```python
from build123d import *

# Parameters (mm, degrees)
SKETCH_1_R          = 1.5
EXTRUDE_1_DEPTH     = 10
CUT_EXTRUDE_2_DEPTH = 10


with BuildPart() as part:
    # 草图1 → 凸台-拉伸1 (new body)
    with BuildSketch(Plane.XY):
        with BuildLine():
            Line((1.5, 19.943670675), (1.5, 25))
            Line((1.5, 25), (-1.5, 25))
            Line((-1.5, 25), (-1.5, 19.943670675))
            ThreePointArc((-1.5, 19.943670675), (-6.180339888, 19.021130326), (-10.509070008, 17.016446385))
            Line((-10.509070008, 17.016446385), (-13.481105816, 21.107102738))
            Line((-13.481105816, 21.107102738), (-15.908156799, 19.343746981))
            Line((-15.908156799, 19.343746981), (-12.936120991, 15.253090628))
            ThreePointArc((-12.936120991, 15.253090628), (-16.180339887, 11.755705046), (-18.504032463, 7.589517943))
            Line((-18.504032463, 7.589517943), (-23.312887416, 9.152009634))
            Line((-23.312887416, 9.152009634), (-24.239938399, 6.298840085))
            Line((-24.239938399, 6.298840085), (-19.431083446, 4.736348394))
            ThreePointArc((-19.431083446, 4.736348394), (-20, 0), (-19.431083446, -4.736348394))
            Line((-19.431083446, -4.736348394), (-24.239938399, -6.298840085))
            Line((-24.239938399, -6.298840085), (-23.312887416, -9.152009634))
            Line((-23.312887416, -9.152009634), (-18.504032463, -7.589517943))
            ThreePointArc((-18.504032463, -7.589517943), (-16.180339887, -11.755705046), (-12.936120991, -15.253090628))
            Line((-12.936120991, -15.253090628), (-15.908156799, -19.343746981))
            Line((-15.908156799, -19.343746981), (-13.481105816, -21.107102738))
            Line((-13.481105816, -21.107102738), (-10.509070008, -17.016446385))
            ThreePointArc((-10.509070008, -17.016446385), (-6.180339887, -19.021130326), (-1.5, -19.943670675))
            Line((-1.5, -19.943670675), (-1.5, -25))
            Line((-1.5, -25), (1.5, -25))
            Line((1.5, -25), (1.5, -19.943670675))
            ThreePointArc((1.5, -19.943670675), (6.180339888, -19.021130326), (10.509070008, -17.016446385))
            Line((10.509070008, -17.016446385), (13.481105816, -21.107102738))
            Line((13.481105816, -21.107102738), (15.908156799, -19.343746981))
            Line((15.908156799, -19.343746981), (12.936120991, -15.253090628))
            ThreePointArc((12.936120991, -15.253090628), (16.180339887, -11.755705046), (18.504032463, -7.589517943))
            Line((18.504032463, -7.589517943), (23.312887416, -9.152009634))
            Line((23.312887416, -9.152009634), (24.239938399, -6.298840085))
            Line((24.239938399, -6.298840085), (19.431083446, -4.736348394))
            ThreePointArc((19.431083446, -4.736348394), (20, 0), (19.431083446, 4.736348394))
            Line((19.431083446, 4.736348394), (24.239938399, 6.298840085))
            Line((24.239938399, 6.298840085), (23.312887416, 9.152009634))
            Line((23.312887416, 9.152009634), (18.504032463, 7.589517943))
            ThreePointArc((18.504032463, 7.589517943), (16.180339887, 11.755705046), (12.936120991, 15.253090628))
            Line((12.936120991, 15.253090628), (15.908156799, 19.343746981))
            Line((15.908156799, 19.343746981), (13.481105816, 21.107102738))
            Line((13.481105816, 21.107102738), (10.509070008, 17.016446385))
            ThreePointArc((10.509070008, 17.016446385), (6.180339887, 19.021130326), (1.5, 19.943670675))
        make_face()
        with Locations((0, 12.5)):
            Circle(SKETCH_1_R, mode=Mode.SUBTRACT)
        with Locations((10.825317547, -6.25)):
            Circle(SKETCH_1_R, mode=Mode.SUBTRACT)
        with Locations((-10.825317547, -6.25)):
            Circle(SKETCH_1_R, mode=Mode.SUBTRACT)
    extrude(amount=EXTRUDE_1_DEPTH)

    # 草图2 → 切除-拉伸2 (cut)
    with BuildSketch(Plane.XY):
        with BuildLine():
            Line((-9.312271895, 3.644391878), (-13.675265955, 6.163367673))
            ThreePointArc((-13.675265955, 6.163367673), (-14.883992786, 1.861923398), (-14.772116295, -2.604722665))
            Line((-14.772116295, -2.604722665), (-17.726539554, -3.125667198))
            ThreePointArc((-17.726539554, -3.125667198), (-15.588457268, 9), (-6.15636258, 16.914467174))
            Line((-6.15636258, 16.914467174), (-5.13030215, 14.095389312))
            ThreePointArc((-5.13030215, 14.095389312), (-9.054469356, 11.958954164), (-12.175265955, 8.761443884))
            Line((-12.175265955, 8.761443884), (-7.812271895, 6.242468089))
            ThreePointArc((-7.812271895, 6.242468089), (0, 10), (7.812271895, 6.242468089))
            Line((7.812271895, 6.242468089), (12.175265955, 8.761443884))
            ThreePointArc((12.175265955, 8.761443884), (9.054469356, 11.958954164), (5.13030215, 14.095389312))
            Line((5.13030215, 14.095389312), (6.15636258, 16.914467174))
            ThreePointArc((6.15636258, 16.914467174), (15.588457268, 9), (17.726539554, -3.125667198))
            Line((17.726539554, -3.125667198), (14.772116295, -2.604722665))
            ThreePointArc((14.772116295, -2.604722665), (14.883992786, 1.861923398), (13.675265955, 6.163367673))
            Line((13.675265955, 6.163367673), (9.312271895, 3.644391878))
            ThreePointArc((9.312271895, 3.644391878), (8.660254038, -5), (1.5, -9.886859967))
            Line((1.5, -9.886859967), (1.5, -14.924811557))
            ThreePointArc((1.5, -14.924811557), (5.829523431, -13.820877562), (9.641814145, -11.490666647))
            Line((9.641814145, -11.490666647), (11.570176974, -13.788799976))
            ThreePointArc((11.570176974, -13.788799976), (0, -18), (-11.570176974, -13.788799976))
            Line((-11.570176974, -13.788799976), (-9.641814145, -11.490666647))
            ThreePointArc((-9.641814145, -11.490666647), (-5.829523431, -13.820877562), (-1.5, -14.924811557))
            Line((-1.5, -14.924811557), (-1.5, -9.886859967))
            ThreePointArc((-1.5, -9.886859967), (-8.660254038, -5), (-9.312271895, 3.644391878))
        make_face()
    extrude(amount=CUT_EXTRUDE_2_DEPTH, mode=Mode.SUBTRACT)


solid = part.part
```
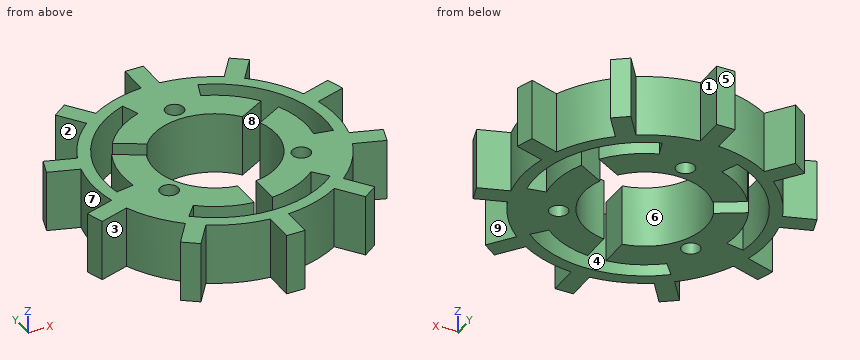
Verification items for the finished model (mm, model axes). Face numbers are marked on the shaded views. A direction names the side the tool comes from. Round coordinates to 2 decimals unless told otherwise and drop trailing zeros. Write each loop counter-clockwise with the first axis right and the second up, starting at its lowest first coordinate (ties: lowest second). Pieces come first, ordered by that corner, then holes. Notation, with made-up numbers: (-28.5, 89) -> (24.5, 89) arc R8 ccw to (24.5, 97) -> close; hole circle Ø10 at (35.5, 48.5). An arc over 180 degrees is marked (long way). Write each question's results on one line, items separated by ' | '. Start each with the question number.
1. Cross-section at C-C (x = 0). Enter the section's corners in (y, z), then the cut area to 3 significant figures.
2. Depth check by flat-ended pin: P1, Ø6, axis at x = -19, z = 6, coming from the -Y side; P2, Ø4, axis at y = 21.5, z = 5.5, coming from the -X side; P3, Ø5.5, axis at y = -12.5, z = 7.5, coming from the +X side; P4, Ø6, axis at x = -4, z = 3, coming from the -Y side. Enter the tip coordinate at first touch or a pass-through.
3. Cross-section at D-D (z = 3.75). Count the separate pieces of the cut face and the enclosed holes in it, then the cut area to 3 significant figures.
4. Set-up check for the marked faces 1, 2, 3, 4 and 5: record each of +Z, -Z, +X, -X, +Y, -Y from which the full face is reachable in a straight line by a thin tool's end or side.
5. Material ranges on probe 1 along X at (y, z) = (-21, 4.5); probe 2 along Y at (x, z) = (12, 4.25); probe 3 along Y at (x, z) = (-2, 3), recorded low to high. Write a range as from..to.
6. Cross-section at A-A (x = -8.5). Enter the section's corners in (y, z).
7. Draft check along X on the marked faces 6, 7, 8 and 9. Enter one of: +X half, -X half, draft (parallel to the pull), parting line (faces both ways), or undercut.
8. Cross-section at B-B (y = -7). Enter the section's corners in (x, z), then the cut area to 3 significant figures.
Solutions:
1) outline: (-25, 0) -> (-18, 0) -> (-18, 10) -> (-25, 10) -> close; (10, 0) -> (11, 0) -> (11, 10) -> (10, 10) -> close; (14, 0) -> (25, 0) -> (25, 10) -> (14, 10) -> close | area: 190 mm2
2) P1: stops at y = -12 | P2: stops at x = -15.69 | P3: stops at x = 17.46 | P4: stops at y = -25
3) separate pieces: 1 | enclosed holes: 4 | area: 819 mm2
4) face 1: +Z, -Z, +Y | face 2: +Z, -Z, -X | face 3: +Z, -Z, -Y | face 4: +Z, -Z | face 5: +Z, -Z, +X, -X, +Y
5) probe 1: x = -13.63..-13.4, -1.5..1.5, 13.4..13.63 | probe 2: y = -19.07..-7.18, -5.32..5.2, 8.66..9, 13.42..19.07 | probe 3: y = -19.9..-17.89, -14.87..-9.8, 9.8..19.9
6) outline: (-18.1, 0) -> (-15.87, 0) -> (-15.87, 10) -> (-18.1, 10) -> close; (-12.36, 0) -> (-5.27, 0) -> (-5.27, 10) -> (-12.36, 10) -> close; (6.64, 0) -> (12.36, 0) -> (12.36, 10) -> (6.64, 10) -> close; (15.87, 0) -> (18.1, 0) -> (18.1, 10) -> (15.87, 10) -> close
7) face 6: undercut | face 7: -X half | face 8: undercut | face 9: +X half
8) outline: (-24.01, 0) -> (-12.12, 0) -> (-12.12, 10) -> (-24.01, 10) -> close; (-9.53, 0) -> (-7.14, 0) -> (-7.14, 10) -> (-9.53, 10) -> close; (7.14, 0) -> (9.53, 0) -> (9.53, 10) -> (7.14, 10) -> close; (12.12, 0) -> (24.01, 0) -> (24.01, 10) -> (12.12, 10) -> close | area: 285 mm2
